```python
from build123d import *

# Parameters (mm, degrees)
SKETCH1_W           = 75
SKETCH1_H           = 50
BOSS_EXTRUDE1_DEPTH = 12
SKETCH2_R           = 4.5
CUT_EXTRUDE1_DEPTH  = 113.445542375
SKETCH3_W           = 30
SKETCH3_H           = 30
CUT_EXTRUDE2_DEPTH  = 4
SKETCH4_W           = 25
SKETCH4_H           = 20
CUT_EXTRUDE3_DEPTH  = 8
FILLET1_R           = 3
SKETCH5_R           = 1.5
CUT_EXTRUDE4_DEPTH  = 113.089250154
SKETCH6_R           = 2.5
CUT_EXTRUDE5_DEPTH  = 113.089250154


with BuildPart() as part:
    # Sketch1 → Boss-Extrude1 (new body)
    with BuildSketch(Plane(origin=(0, 0, 0), x_dir=(1, 0, 0), z_dir=(0, 1, 0))):
        with Locations((37.5, 25)):
            Rectangle(SKETCH1_W, SKETCH1_H)
        with BuildLine():
            Line((75, 0), (75, 50))
            ThreePointArc((75, 50), (100, 25), (75, 0))
        make_face()
        with BuildLine():
            Line((0, 0), (0, 50))
            ThreePointArc((0, 50), (-25, 25), (0, 0))
        make_face()
    extrude(amount=BOSS_EXTRUDE1_DEPTH)

    # Sketch2 → Cut-Extrude1 (cut, through all)
    with BuildSketch(Plane(origin=(0, 12, 0), x_dir=(1, 0, 0), z_dir=(0, 1, 0))):
        with Locations(Location((-10, 25, 0), (0, 0, 270))):
            Circle(SKETCH2_R)
        with Locations(Location((85, 25, 0), (0, 0, 90))):
            Circle(SKETCH2_R)
    extrude(amount=-CUT_EXTRUDE1_DEPTH, mode=Mode.SUBTRACT)

    # Sketch3 → Cut-Extrude2 (cut)
    with BuildSketch(Plane(origin=(0, 12, 0), x_dir=(1, 0, 0), z_dir=(0, 1, 0))):
        with Locations((24.041436108, 25)):
            Rectangle(SKETCH3_W, SKETCH3_H)
    extrude(amount=-CUT_EXTRUDE2_DEPTH, mode=Mode.SUBTRACT)

    # Sketch4 → Cut-Extrude3 (cut)
    with BuildSketch(Plane(origin=(0, 12, 0), x_dir=(1, 0, 0), z_dir=(0, 1, 0))):
        with Locations((51.541436108, 25)):
            Rectangle(SKETCH4_W, SKETCH4_H)
    extrude(amount=-CUT_EXTRUDE3_DEPTH, mode=Mode.SUBTRACT)

    # Fillet1
    fillet1_edges = [part.edges().sort_by_distance(p)[0] for p in [
        (9.041436108, 10, -10),
        (9.041436108, 10, -40),
        (39.041436108, 10, -40),
        (39.041436108, 10, -10),
        (64.041436108, 8, -15),
        (39.041436108, 6, -15),
        (39.041436108, 6, -35),
        (64.041436108, 8, -35),
    ]]
    fillet(fillet1_edges, radius=FILLET1_R)

    # Sketch5 → Cut-Extrude4 (cut, through all)
    with BuildSketch(Plane(origin=(0, 4, 0), x_dir=(1, 0, 0), z_dir=(0, 1, 0))):
        with Locations(Location((51.541436108, 25, 0), (0, 0, 270))):
            Circle(SKETCH5_R)
    extrude(amount=-CUT_EXTRUDE4_DEPTH, mode=Mode.SUBTRACT)

    # Sketch6 → Cut-Extrude5 (cut, through all)
    with BuildSketch(Plane(origin=(0, 8, 0), x_dir=(1, 0, 0), z_dir=(0, 1, 0))):
        with Locations(Location((16.541436108, 25, 0), (0, 0, 270))):
            Circle(SKETCH6_R)
        with Locations(Location((31.541436108, 25, 0), (0, 0, 270))):
            Circle(SKETCH6_R)
    extrude(amount=-CUT_EXTRUDE5_DEPTH, mode=Mode.SUBTRACT)


solid = part.part
```
The listing builds one solid part. Answer for the finished solid, in the listing's coordinates (mm). A direction names the side the tool comes from. Coordinates: 2 decimals unless noted, no trailing zeros. Loops run counter-clockwise (first coordinate to the right, second up) from the corner with the lowest first, then second, coordinate; pieces in that order, holes last. Notation, with made-up numbers: (35, -27.75) -> (90, -27.75) arc R30 cw to (90, -1.75) -> close; hole circle Ø11 at (-21, -28.75). An arc over 180 degrees is marked (long way). Use one line per item in the form item = value. Start each with the question number.
Item 1: The part is cut by section B-B on y = 10. Determine the outline of the cut face in (x, z).
Item 2: Consider L1, parallel to X at y = 5.5, z = -25; L2, parallel to X at y = 2.5, z = -25; L3, parallel to Z at x = 27, y = 11.5. Determine where each line is inside the solid, lowest interval first. Write a range as [from, to].
Item 3: The part is cut by section D-D on y = 2.25. Determine the outline of the cut face in (x, z).
Item 4: A tool of negligible diameter and unlimited length cuts with its end or side. For faces 5 (the face through (50.63, 2.03, -26.19)), 6 (the face through (63.186, 7.944, -34.098)), from which of +Z, -Z, +X, -X, +Y, -Y can it reach the whole face along a straight path? Write none if from no direction.
Item 5: The part is cut by section A-A on z = -25. Count the separate pieces of the cut face and the enclosed holes in it, then the cut area to 3 significant figures.
Item 6: Flat-ended cylindrical pins translate along their axes: pin 1 Ø0.6 at (y, z) = (11, -35.5) entering from -X; pin 2 Ø2 at (x, z) = (52, -18) entering from +Y; pin 3 Ø6 at (x, z) = (16.54, -25) entering from +Y. Find the tip coordinate at first contact, or state that the pin passes through.
Item 7: The part is cut by section C-C on x = 46. Determine the outline of the cut face in (y, z).
Item 8: The mould has two halves that part along Z. Classify faces 1 (the face through (25, 8, -25)), 2 (the face through (37, 12, -9)), 3 (the face through (37, 6, -50)), 4 (the face through (99.994, 5.916, -25.55)): released by +Z, released by -Z, zero draft, split by the parting line, or undercut.
Answer key:
q1.outline = (0, -50) -> (75, -50) arc R25 ccw to (75, 0) -> (0, 0) arc R25 ccw to start; hole circle Ø9 at (-10, -25); hole (9.04, -37) arc R3 ccw to (12.04, -40) -> (36.04, -40) arc R3 ccw to (39.04, -37) -> (39.04, -35) -> (61.04, -35) arc R3 ccw to (64.04, -32) -> (64.04, -18) arc R3 ccw to (61.04, -15) -> (39.04, -15) -> (39.04, -13) arc R3 ccw to (36.04, -10) -> (12.04, -10) arc R3 ccw to (9.04, -13) -> close; hole circle Ø9 at (85, -25)
q2.L1 = [-25, -14.5], [-5.5, 14.04], [19.04, 29.04], [34.04, 39.04], [64.04, 80.5], [89.5, 100]
q2.L2 = [-25, -14.5], [-5.5, 14.04], [19.04, 29.04], [34.04, 50.04], [53.04, 80.5], [89.5, 100]
q2.L3 = [-50, -40], [-10, 0]
q3.outline = (0, -50) -> (75, -50) arc R25 ccw to (75, 0) -> (0, 0) arc R25 ccw to start; hole circle Ø9 at (-10, -25); hole circle Ø5 at (16.54, -25); hole circle Ø5 at (31.54, -25); hole circle Ø3 at (51.54, -25); hole circle Ø9 at (85, -25)
q4.face_5 = +Y, -Y
q4.face_6 = +Y
q5.separate_pieces = 6
q5.enclosed_holes = 0
q5.area = 872 mm2
q6.pin_1 = -22.82
q6.pin_2 = 4
q6.pin_3 = 8
q7.outline = (0, -50) -> (12, -50) -> (12, -35) -> (4, -35) -> (4, -15) -> (12, -15) -> (12, 0) -> (0, 0) -> close
q8.face_1 = undercut
q8.face_2 = zero draft
q8.face_3 = released by -Z
q8.face_4 = split by the parting line
